Could you check a few things on this model? Use its own coordinates, in mm. Give positions to 0.01 mm unless a question says otherwise; leave off trailing zeros. Order: outer loops, then holes, each group sorted by start corner. A loop starts at its lowest first (then second) coordinate and runs counter-clockwise, first axis right, second up.
Autodesk Inventor part; units mm, degrees
ref_plane "YZ Plane" through (0, 0, 0) normal (1, 0, 0) x (0, 1, 0)
ref_plane "XZ Plane" through (0, 0, 0) normal (0, 1, 0) x (-1, 0, 0)
ref_plane "XY Plane" through (0, 0, 0) normal (0, 0, 1) x (1, 0, 0)
sketch "Sketch1" plane through (0, 0, 0) normal (0, 0, 1) x (1, 0, 0)
  circle A0 centre (0, 0) radius 35
  dimension "d0" = 70
extrude "Extrusion1" add sketch "Sketch1" along normal blind 2
sketch "Sketch2" plane through (0, 0, 2) normal (0, 0, 1) x (1, 0, 0)
  circle A0 centre (0, 0) radius 36
  dimension "d3" = 72
extrude "Extrusion2" add sketch "Sketch2" along normal blind 21
chamfer "Chamfer1" distance 3 angle 45 1 edges at (-36, 0, 23)
properties part number "LIdar_p2"
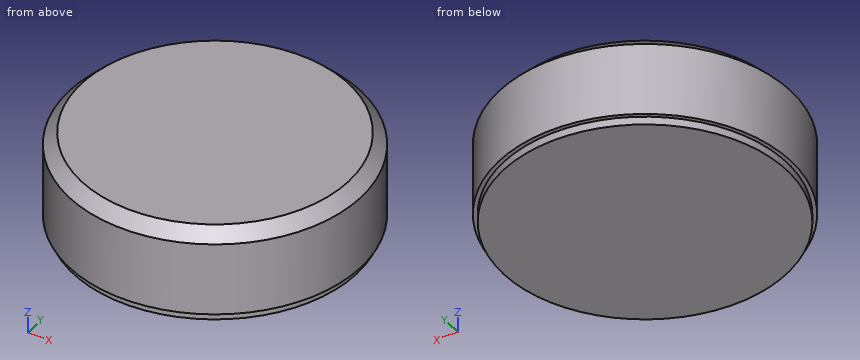
Item 1: Imagine slicing it at A-A on z = 16. List the corners of the cut face in (x, y) for me.
Findings:
outline: circle Ø72 at (0, 0)
Item 2: Please list where these lines run through material, in increasing order: line 1 along X through (y, z) = (13, 21); line 2 along X through (y, z) = (-9, 6.75); line 3 along Y through (x, z) = (20.5, 11).
Findings:
line 1: x = -32.5 to 32.5
line 2: x = -34.86 to 34.86
line 3: y = -29.59 to 29.59
Item 3: For pin 1 (10 mm diameter, centred on x = 15, z = 14, fed in from -Y); pin 2 (5 mm diameter, centred on x = -29, z = 12.5, fed in from -Y); pin 3 (8 mm diameter, centred on y = -17.5, z = 20.5, fed in from +X), each with a flat end and sliding along its axis, tell me the tip position at first contact or that it passes through.
Findings:
pin 1: stops at y = -34.58
pin 2: stops at y = -24.37
pin 3: stops at x = 33.36
